Could you check a few things on this model? Use its own coordinates, in mm. Face numbers are marked on the shaded views. A direction names the side the tool comes from. Coordinates: 2 decimals unless noted, no trailing zeros. Order: outer loops, then holes, each group sorted by start corner. A loop starts at its lowest first (then second) coordinate and runs counter-clockwise, first axis right, second up. Notation, with made-up numbers: (27.5, 3.5) -> (42.5, 3.5) arc R36 cw to (42.5, 40.5) -> close; hole circle Ø9 at (43.5, 52.25). An arc over 180 degrees is marked (long way). Put each result on its own line as item: value. Start each with the question number.
Q1. Will these pins go through, and if not, where does the flat tip stop? pin 1 (1 mm diameter, centred on x = -3.5, z = 16.5, fed in from -Y); pin 2 (2 mm diameter, centred on y = -3.5, z = 4.5, fed in from -X); pin 3 (3.5 mm diameter, centred on y = 0, z = 14, fed in from -X).
Q2. If we section it at D-D (x = 6.25): Please give me the cut outline in (y, z).
Q3. Please list where these lines run through material, in increasing order: line 1 along Z through (x, y) = (5.05, 0); line 2 along Y through (x, z) = (0, 6.5); line 3 along Y through (x, z) = (3.9, 14).
Q4. If we section it at C-C (z = 10.25): Please give me the cut outline in (x, y).
Q5. If we section it at A-A (x = 0): Please give me the cut outline in (y, z).
Q6. We'd pull the mould along X, two halves only. Please class the marked faces 3, 4, 5 and 6: +X half, -X half, draft (parallel to the pull), parting line (faces both ways), or undercut.
Q7. For the marked faces 1 and 2, which set-ups out of +Z, -Z, +X, -X, +Y, -Y let a thin tool reach every point of the face, with its end or its side?
from build123d import *

# Parameters (mm, degrees)
F0_R     = 7.5
F0_R_2   = 3
F1_DEPTH = 18.5
F2_START = 2
F0_R_3   = 8.5
F2_DEPTH = 9
F3_R     = 1.5
F4_DEPTH = 8.501
F5_R     = 1.5
F6_DEPTH = 8.501


with BuildPart() as f1:
    # F0 (on Top) → F1 (new body)
    with BuildSketch(Plane.XY):
        Circle(F0_R)
        Circle(F0_R_2, mode=Mode.SUBTRACT)
    extrude(amount=F1_DEPTH)

    # F0 (on Top) → F2 (join)
    with BuildSketch(Plane.XY.offset(F2_START)):
        Circle(F0_R_3)
        Circle(F0_R, mode=Mode.SUBTRACT)
    extrude(amount=F2_DEPTH)

    # F3 (on Right) → F4 (cut, through all)
    with BuildSketch(Plane.YZ):
        with Locations((0, 14)):
            Circle(F3_R)
    extrude(amount=F4_DEPTH, mode=Mode.SUBTRACT)

    # F5 (on Front) → F6 (cut, through all)
    with BuildSketch(Plane.XZ):
        with Locations((0, 14)):
            Circle(F5_R)
    extrude(amount=-F6_DEPTH, mode=Mode.SUBTRACT)


solid = f1.part
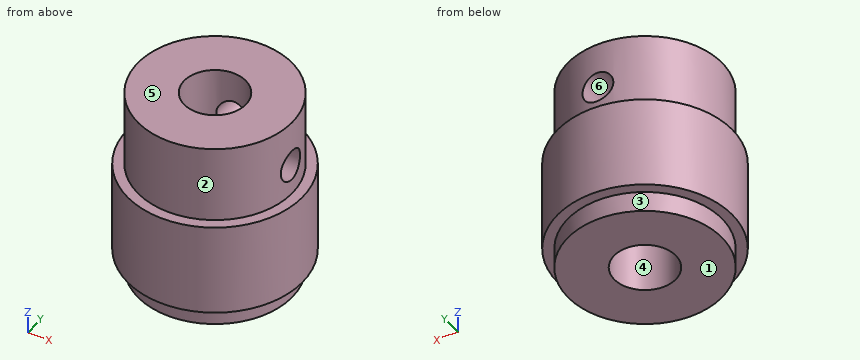
The answers:
1. pin 1: y = -6.87
1. pin 2: x = -8.12
1. pin 3: x = -7.5
2. outline: (-5.76, 2) -> (-4.15, 2) -> (-4.15, 0) -> (4.15, 0) -> (4.15, 2) -> (5.76, 2) -> (5.76, 11) -> (4.15, 11) -> (4.15, 18.5) -> (-4.15, 18.5) -> (-4.15, 11) -> (-5.76, 11) -> close; hole circle Ø3 at (0, 14)
3. line 1: 0 to 12.5, 15.5 to 18.5
3. line 2: -8.5 to -3, 3 to 8.5
3. line 3: -6.41 to -1.5, 1.5 to 6.41
4. outline: circle Ø17 at (0, 0); hole circle Ø6 at (0, 0)
5. outline: (-8.5, 2) -> (-7.5, 2) -> (-7.5, 0) -> (-3, 0) -> (-3, 18.5) -> (-7.5, 18.5) -> (-7.5, 11) -> (-8.5, 11) -> close; (3, 0) -> (7.5, 0) -> (7.5, 2) -> (8.5, 2) -> (8.5, 11) -> (7.5, 11) -> (7.5, 12.5) -> (3, 12.5) -> close; (3, 15.5) -> (7.5, 15.5) -> (7.5, 18.5) -> (3, 18.5) -> close
6. face 3: parting line
6. face 4: undercut
6. face 5: draft
6. face 6: undercut
7. face 1: -Z, +X, -X, +Y, -Y
7. face 2: +Z
